Check sheet for the modelled part. Datum: model origin and axes. Units: mm. A direction names the side the tool comes from. Round coordinates to 2 decimals unless told otherwise and drop trailing zeros. Write each loop counter-clockwise with the first axis right and the second up, starting at its lowest first coordinate (ties: lowest second). Pieces come first, ordered by that corner, then holes. Notation, with made-up numbers: M 8,8 L 38,8 A21 cw 38,47 Z; hole C 31,-21 d3. An arc over 180 degrees is marked long. One line per item, written item: value.
from build123d import *

# Parameters (mm, degrees)
SKETCH1_W           = 24.892
SKETCH1_H           = 7.874
BOSS_EXTRUDE1_DEPTH = 2.286
SKETCH2_R           = 4
BOSS_EXTRUDE2_DEPTH = 8.29
SKETCH3_R           = 1.825
CUT_EXTRUDE1_DEPTH  = 8.29
SKETCH4_R           = 4
BOSS_EXTRUDE3_DEPTH = 8.29
SKETCH5_R           = 1.825
CUT_EXTRUDE2_DEPTH  = 8.29
SKETCH7_W           = 2.286
SKETCH7_H           = 24
BOSS_EXTRUDE4_DEPTH = 24.892


with BuildPart() as part:
    # Sketch1 → Boss-Extrude1 (new body)
    with BuildSketch(Plane.XY):
        with Locations((-11.83196875, 3.65678125)):
            Rectangle(SKETCH1_W, SKETCH1_H)
    extrude(amount=BOSS_EXTRUDE1_DEPTH)

    # Sketch4 → Boss-Extrude3 (add)
    with BuildSketch(Plane.ZY.offset(24.27796875)):
        with Locations(Location((1.143, 11.09378125, 0), (0, 0, 90))):
            Circle(SKETCH4_R)
    extrude(amount=-BOSS_EXTRUDE3_DEPTH)

    # Sketch5 → Cut-Extrude2 (cut)
    with BuildSketch(Plane.ZY.offset(24.27796875)):
        with Locations(Location((1.143, 11.09378125, 0), (0, 0, 90))):
            Circle(SKETCH5_R)
    extrude(amount=-CUT_EXTRUDE2_DEPTH, mode=Mode.SUBTRACT)



with BuildPart() as body_2:
    # Sketch2 → Boss-Extrude2 (new body)
    with BuildSketch(Plane(origin=(0.61403125, 0, 0), x_dir=(0, 0, -1), z_dir=(1, 0, 0))):
        with Locations(Location((-1.143, 11.09378125, 0), (0, 0, 90))):
            Circle(SKETCH2_R)
    extrude(amount=-BOSS_EXTRUDE2_DEPTH)

    # Sketch3 → Cut-Extrude1 (cut)
    with BuildSketch(Plane(origin=(0.61403125, 0, 0), x_dir=(0, 0, -1), z_dir=(1, 0, 0))):
        with Locations(Location((-1.143, 11.09378125, 0), (0, 0, 90))):
            Circle(SKETCH3_R)
    extrude(amount=-CUT_EXTRUDE1_DEPTH, mode=Mode.SUBTRACT)


with BuildPart() as part_1:
    add(part.part)

    add(body_2.part)  # Boss-Extrude4 merges body 2
    # Sketch7 → Boss-Extrude4 (add)
    with BuildSketch(Plane.ZY.offset(24.27796875)):
        with Locations((1.143, -4.739435545)):
            Rectangle(SKETCH7_W, SKETCH7_H)
    extrude(amount=-BOSS_EXTRUDE4_DEPTH)


solid = part_1.part
Q1. Sectioned sample at B-B on y = 11. Enter the section's corners in (x, z), and give its area (3 significant figures).
Completed:
outline: M -24.28,-2.86 L -15.99,-2.86 L -15.99,-0.68 L -24.28,-0.68 Z; M -24.28,2.97 L -15.99,2.97 L -15.99,5.14 L -24.28,5.14 Z; M -7.68,-2.86 L 0.61,-2.86 L 0.61,-0.68 L -7.68,-0.68 Z; M -7.68,2.97 L 0.61,2.97 L 0.61,5.14 L -7.68,5.14 Z
area: 72.2 mm^2
Q2. Depth check by flat-ended pin: P1, Ø2, axis at x = -2.5, y = -6.5, coming from the -Z side; P2, Ø2, axis at y = 11.09, z = 1.14, coming from the +X side; P3, Ø1.1, axis at x = -12.5, z = 1, coming from the +Y side; P4, Ø1, axis at x = -18.5, y = 3, coming from the +Z side. Enter the tip coordinate at first touch or a pass-through.
Completed:
P1: z = 0
P2: through
P3: y = 7.59
P4: z = 2.29
Q3. Sectioned sample at C-C on x = -11. Enter the section's corners in (y, z), and give its area (3 significant figures).
Completed:
outline: M -16.74,0 L 7.59,0 L 7.59,2.29 L -16.74,2.29 Z
area: 55.6 mm^2
Q4. Access from +Z, -Z, +X, -X, +Y, -Y to the whole of each face (thin tool, end or side, straight path). Record for faces 4 (the flat face through (-12, -16.739, 1)), 5 (the flat face through (-12, 7.594, 1)).
Completed:
face 4: +Z, -Z, +X, -X, -Y
face 5: +Z, -Z, +Y
Q5. Draft check along Y on faces 1 (the flat face through (-12, -5, 2.286)), 2 (the cylindrical face through (-3.47, 15.09, 0.98)), 3 (the cylindrical face through (-20.19, 9.27, 1.06)). Enter one of: pulls with the +Y half, pulls with the -Y half, needs draft (parallel to the pull), parting line crosses it, or undercut.
Completed:
face 1: needs draft
face 2: parting line crosses it
face 3: undercut
Q6. Sectioned sample at A-A on z = -1.25. Enter the section's corners in (x, y), and give its area (3 significant figures).
Completed:
outline: M -24.28,7.89 L -15.99,7.89 L -15.99,14.3 L -24.28,14.3 Z; M -7.68,7.89 L 0.61,7.89 L 0.61,14.3 L -7.68,14.3 Z
area: 106 mm^2
Q7. Scan lines: line 1 (X direction, y = 9, z = -1); line 2 (Z direction, x = -10.75, y = -1.5); line 3 (Y direction, x = -0.25, z = 2). Record each from-to range of solid material in increasing order. Write a range as [from, to].
Completed:
line 1: [-24.28, -15.99], [-7.68, 0.61]
line 2: [0, 2.29]
line 3: [-16.74, 9.48], [12.71, 15]
Q8. Sectioned sample at D-D on y = 1. Enter the section's corners in (x, z), and give its area (3 significant figures).
Completed:
outline: M -24.28,0 L 0.61,0 L 0.61,2.29 L -24.28,2.29 Z
area: 56.9 mm^2
